Check sheet for the modelled part. Datum: model origin and axes. Units: mm. A direction names the side the tool comes from. Round coordinates to 2 decimals unless told otherwise and drop trailing zeros. Write each loop counter-clockwise with the first axis right and the second up, starting at its lowest first coordinate (ties: lowest second). Pieces come first, ordered by that corner, then holes. Notation, with made-up numbers: (4, 71) -> (41, 71) arc R4 ccw to (41, 77) -> close; hole circle Ø3 at (-1.5, -30.5). An arc over 180 degrees is marked (long way). Put each result on its own line as item: value. Start each with the question number.
from build123d import *

# Parameters (mm, degrees)
SKETCH1_R           = 2
SKETCH1_R_2         = 1.5875
SKETCH1_W           = 5
SKETCH1_H           = 60
BOSS_EXTRUDE1_DEPTH = 1.5875
FILLET1_R           = 20


with BuildPart() as part:
    # Sketch1 → Boss-Extrude1 (new body, symmetric)
    with BuildSketch(Plane.XY):
        Polygon((-50, -145), (50, -145), (50, -52), (47, -52), (47, -57), (40, -57), (40, -45), (47, -45), (47, -50), (50, -50), (50, 185), (-50, 185), align=None)
        with Locations((-26.5, -129.5)):
            Circle(SKETCH1_R, mode=Mode.SUBTRACT)
        with Locations((-45, -75)):
            Circle(SKETCH1_R_2, mode=Mode.SUBTRACT)
        with BuildLine():
            Line((15, -77.5), (-15, -77.5))
            ThreePointArc((-15, -77.5), (-22.5, -70), (-15, -62.5))
            Line((-15, -62.5), (15, -62.5))
            ThreePointArc((15, -62.5), (22.5, -70), (15, -77.5))
        make_face(mode=Mode.SUBTRACT)
        with Locations((-37.5, -7.531680382)):
            Rectangle(SKETCH1_W, SKETCH1_H, mode=Mode.SUBTRACT)
        with Locations((26.5, -129.5)):
            Circle(SKETCH1_R, mode=Mode.SUBTRACT)
        with Locations((45, -75)):
            Circle(SKETCH1_R_2, mode=Mode.SUBTRACT)
        with Locations((37.5, -7.531680382)):
            Rectangle(SKETCH1_W, SKETCH1_H, mode=Mode.SUBTRACT)
        with BuildLine():
            ThreePointArc((-15, 62.5), (-22.5, 70), (-15, 77.5))
            Line((-15, 77.5), (15, 77.5))
            ThreePointArc((15, 77.5), (22.5, 70), (15, 62.5))
            Line((15, 62.5), (-15, 62.5))
        make_face(mode=Mode.SUBTRACT)
        with Locations((-12, 100)):
            Circle(SKETCH1_R_2, mode=Mode.SUBTRACT)
        with Locations((-26.5, 129.5)):
            Circle(SKETCH1_R, mode=Mode.SUBTRACT)
        with Locations((12, 100)):
            Circle(SKETCH1_R_2, mode=Mode.SUBTRACT)
        with Locations((26.5, 129.5)):
            Circle(SKETCH1_R, mode=Mode.SUBTRACT)
        with Locations((20, 179)):
            Circle(SKETCH1_R_2, mode=Mode.SUBTRACT)
        with Locations((-20, 179)):
            Circle(SKETCH1_R_2, mode=Mode.SUBTRACT)
    extrude(amount=BOSS_EXTRUDE1_DEPTH, both=True)

    # Fillet1
    fillet1_edges = [part.edges().sort_by_distance(p)[0] for p in [
        (-50, 185, 0),
        (50, 185, 0),
        (-50, -145, 0),
        (50, -145, 0),
    ]]
    fillet(fillet1_edges, radius=FILLET1_R)


solid = part.part
1. Draft check along Y on faces 1 (the cylindrical face through (43.986, -139.297, 0.022)), 2 (the cylindrical face through (22.5, 70.16, 0.02)), 3 (the flat face through (-1, 22, 1.588)). Enter one of: released by +Y, released by -Y, zero draft, split by the parting line, or undercut.
2. Gauge pin test, flat ends, axial feed: P1, Ø1, axis at x = 37.5, z = 0.5, coming from the -Y side (3 decimals); P2, Ø2.5, axis at x = -26.5, y = 129.5, coming from the +Z side. Record the tip position at first contact, or that the pin passes through.
3. Section check C-C, the plane z = 0.85. Give the number of separate pieces and of enclosed holes in the cut face, then the cut area to 3 significant figures.
4. Section check A-A, the plane y = -11. Enter the section's corners in (x, z), then the cut area to 3 significant figures.
5. Section check B-B, the plane y = -70. Enter the section's corners in (x, z), then the cut area to 3 significant figures.
6. Access from +Z, -Z, +X, -X, +Y, -Y to the whole of each face (thin tool, end or side, straight path). Record for faces 4 (the cylindrical face through (-44.297, 178.986, -0.022)), 5 (the cylindrical face through (22.5, -69.84, 0.02)).
7. Material ranges on L1, parallel to X at y = -26, z = -0.4; L2, parallel to Y at x = -3, z = -0.45; L3, parallel to Y at x = -26.5, z = -0.65, recorded low to high. Write a range as [from, to].
Reply:
1. face 1: released by -Y
1. face 2: undercut
1. face 3: zero draft
2. P1: stops at y = -143.735
2. P2: passes through
3. separate pieces: 1
3. enclosed holes: 14
3. area: 30,600 mm2
4. outline: (-50, -1.59) -> (-40, -1.59) -> (-40, 1.59) -> (-50, 1.59) -> close; (-35, -1.59) -> (35, -1.59) -> (35, 1.59) -> (-35, 1.59) -> close; (40, -1.59) -> (50, -1.59) -> (50, 1.59) -> (40, 1.59) -> close
4. area: 286 mm2
5. outline: (-50, -1.59) -> (-22.5, -1.59) -> (-22.5, 1.59) -> (-50, 1.59) -> close; (22.5, -1.59) -> (50, -1.59) -> (50, 1.59) -> (22.5, 1.59) -> close
5. area: 175 mm2
6. face 4: +Z, -Z, -X, +Y
6. face 5: +Z, -Z
7. L1: x = [-50, -40], [-35, 35], [40, 50]
7. L2: y = [-145, -77.5], [-62.5, 62.5], [77.5, 185]
7. L3: y = [-145, -131.5], [-127.5, 127.5], [131.5, 185]
